Model file for the job. Use its own axes, mm. A direction names the side the tool comes from. Coordinates: 2 decimals unless noted, no trailing zeros. Return JSON: item names as keys, results as strings.
```python
from build123d import *

# Parameters (mm, degrees)
F3_W     = 4
F3_H     = 13.1636379468
F4_DEPTH = 10.7897276517


with BuildPart() as f2:
    # F1 (on Front) → F2 (revolve)
    with BuildSketch(Plane.XZ):
        with BuildLine():
            ThreePointArc((2, 9.5173232257), (3.7962324027, 4.9229765601), (4.1105155833, 0))
            Line((4.1105155833, 0), (6.425, 0))
            Line((6.425, 0), (7.625, 0))
            Line((7.625, 0), (7.625, 5.8279288933))
            Line((7.625, 5.8279288933), (10.7887275517, 5.8279288933))
            ThreePointArc((10.7887275517, 5.8279288933), (8.2404077135, 10.0788924102), (3.5738223232, 11.7485048249))
            Line((3.5738223232, 11.7485048249), (2, 11.7485048249))
            Line((2, 11.7485048249), (2, 9.5173232257))
        make_face()
    revolve(axis=Axis((0, 0, 0), (0, 0, 1)))

    # F3 (on Right) → F4 (cut, through all)
    with BuildSketch(Plane.YZ):
        with Locations((-0.6494129193, 5.3884481313)):
            Rectangle(F3_W, F3_H)
    extrude(amount=-F4_DEPTH, mode=Mode.SUBTRACT)


solid = f2.part
```
Item 1: Pull direction Y, two halves, no side cores. Call faces 1 (the cylindrical face through (7.616, 0.367, 2.955)), 2 (the flat face through (-6, 1.351, 6)), 3 (the flat face through (4, -3, 0)), 4 (the cylindrical face through (1.852, 0.755, 10.617)): +Y half, -Y half, draft (parallel to the pull), parting line (faces both ways), or undercut.
Check result:
{"face 1": "parting line", "face 2": "undercut", "face 3": "draft", "face 4": "undercut"}
Item 2: 3-axis set-ups, long thin cutter, end or side, ignore diameter. For faces 5 (the flat face through (7.4, 2.5, 5.828)), 6 (the flat face through (-5, -2.649, 7)), 7 (the flat face through (2, 2, 11.749)): which of +Z, -Z, +X, -X, +Y, -Y reach the whole face in a straight line?
Check result:
{"face 5": "-Z", "face 6": "+Z, -Z, -X", "face 7": "+Z, +X, -X, +Y, -Y"}
Item 3: Wall check: line 1 (Y direction, x = 2.75, z = 3.5); line 2 (Y direction, x = -3.5, z = 6); line 3 (Z direction, x = -2.5, y = 8). Give the ranges that are in metal, low to high.
Check result:
{"line 1": "y = -7.11 to -2.97, 2.97 to 7.11", "line 2": "y = -10.17 to -2.65, 1.35 to 10.17", "line 3": "z = 5.83 to 9.96"}
Item 4: Drop flat-ended pins along their axis: pin 1 Ø1 at (y, z) = (-6, 5) entering from +X; pin 2 Ø1 at (x, y) = (-5, -7.5) entering from +Z; pin 3 Ø0.7 at (y, z) = (-2, 10.5) entering from -X. Give the stop position or say it passes through.
Check result:
{"pin 1": "stops at x = 5.28", "pin 2": "stops at z = 9.84", "pin 3": "stops at x = 0"}
